Check sheet for the modelled part. Datum: model origin and axes. Units: mm. Round coordinates to 2 decimals unless told otherwise and drop trailing zeros. Write each loop counter-clockwise with the first axis right and the second up, starting at its lowest first coordinate (ties: lowest second). Pieces come first, ordered by that corner, then holes.
Item 1: Release check for a two-part mould opening along Y. For faces 1 (the cylindrical face through (-17.871, -117.482, 10.14)), 2 (the cylindrical face through (-1.302, 109.915, 10.14)), 3 (the flat face through (0, 2, 20)) record: +Y half, -Y half, draft (parallel to the pull), parting line (faces both ways), or undercut.
Item 2: Material ranges on line 1 (Y direction, x = 0, z = 6); line 2 (Y direction, x = -1.5, z = 9.5); line 3 (Y direction, x = 15.5, z = 1), recorded low to high.
Item 3: Cross-section at A-A on z = 6.5. Count the separate pieces of the cut face and the enclosed holes in it, plus the area to 3 significant figures.
Item 4: Go/stop test with flat-tipped pins: pin 1 Ø3 at (x, z) = (-14, 9) entering from +Y; pin 2 Ø18 at (x, y) = (0, -100) entering from -Z; pin 3 Ø1 at (x, z) = (15, 13) entering from +Y; pin 4 Ø5 at (x, z) = (6.5, 17) entering from -Y. Record where each tip stops, or that it passes through.
Item 5: Cross-section at B-B on x = -21. Enter the section's corners in (y, z).
from build123d import *

# Parameters (mm, degrees)
ESQUISSE1_W             = 50
ESQUISSE1_H             = 250
BOSS_EXTRU_1_DEPTH      = 20
ENL_V_MAT_EXTRU_1_REACH = 131.035
ESQUISSE2_R             = 10
CONG_1_R                = 25


with BuildPart() as part:
    # Esquisse1 → Boss.-Extru.1 (new body)
    with BuildSketch(Plane.XY):
        Rectangle(ESQUISSE1_W, ESQUISSE1_H)
    extrude(amount=BOSS_EXTRU_1_DEPTH)

    # Esquisse2 → Enlèv. mat.-Extru.1 (cut, up to next)
    with BuildSketch(Plane.XY.offset(20), mode=Mode.PRIVATE) as enl_v_mat_extru_1_sk1:
        with Locations((0, -100)):
            Circle(ESQUISSE2_R)
    enl_v_mat_extru_1_tool1 = extrude(enl_v_mat_extru_1_sk1.sketch, amount=-ENL_V_MAT_EXTRU_1_REACH, mode=Mode.PRIVATE) & part.part
    # Esquisse2 → Enlèv. mat.-Extru.1 (cut, up to next)
    with BuildSketch(Plane.XY.offset(20), mode=Mode.PRIVATE) as enl_v_mat_extru_1_sk2:
        with Locations((0, 100)):
            Circle(ESQUISSE2_R)
    enl_v_mat_extru_1_tool2 = extrude(enl_v_mat_extru_1_sk2.sketch, amount=-ENL_V_MAT_EXTRU_1_REACH, mode=Mode.PRIVATE) & part.part
    add(enl_v_mat_extru_1_tool1.solids().sort_by_distance((0, -100, 20))[0], mode=Mode.SUBTRACT)
    add(enl_v_mat_extru_1_tool2.solids().sort_by_distance((0, 100, 20))[0], mode=Mode.SUBTRACT)

    # Congé1
    cong_1_edges = [part.edges().sort_by_distance(p)[0] for p in [
        (-25, -125, 10),
        (25, -125, 10),
        (-25, 125, 10),
        (25, 125, 10),
    ]]
    fillet(cong_1_edges, radius=CONG_1_R - 0.0001)  # a hair under: the kernel refuses the full size


solid = part.part
Response values:
1. face 1: -Y half
1. face 2: undercut
1. face 3: draft
2. line 1: y = -125 to -110, -90 to 90, 110 to 125
2. line 2: y = -124.95 to -109.89, -90.11 to 90.11, 109.89 to 124.95
2. line 3: y = -119.62 to 119.62
3. separate pieces: 1
3. enclosed holes: 2
3. area: 11,300 mm2
4. pin 1: stops at y = 121.65
4. pin 2: passes through
4. pin 3: stops at y = 120.37
4. pin 4: stops at y = -124.68
5. outline: (-113.56, 0) - (113.56, 0) - (113.56, 20) - (-113.56, 20) - close
